Input: part model. Units: mm. Frame: model coordinates. Give positions to 0.01 mm unless a question says otherwise; leave off trailing zeros. Write each loop counter-clockwise with the first axis right and the second up, starting at its lowest first coordinate (ties: lowest second). Pieces come first, ordered by that corner, then holes. Notation, with made-up numbers: (39, -35.75) -> (82, -35.75) arc R24 cw to (82, -3.75) -> close; hole circle Ø1 at (-15.5, -16.5). An arc over 180 degrees is marked (long way). Answer as a JSON object with one key per item and string values. Group by question number.
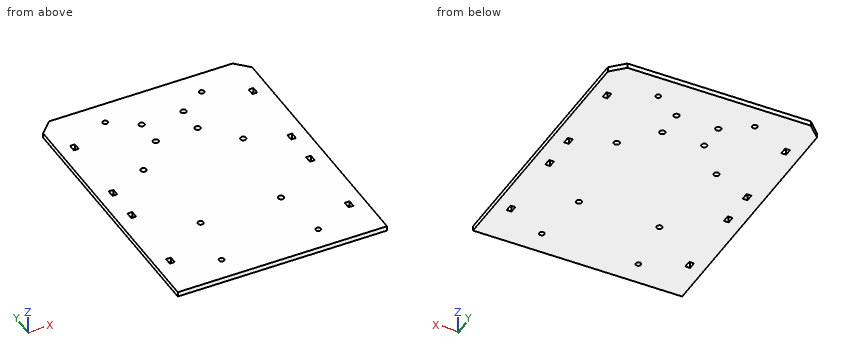
from build123d import *

# Parameters (mm, degrees)
SKETCH_1_R      = 1.6
SKETCH_1_R_2    = 1.75
SKETCH_1_W      = 3
SKETCH_1_H      = 4.6
EXTRUDE_1_DEPTH = 3


with BuildPart() as part:
    # ｽｹｯﾁ1 → ﾎﾞｽ - 押し出し1 (new body)
    with BuildSketch(Plane.XY):
        Polygon((0, 162), (8, 170), (122, 170), (130, 162), (130, 0), (0, 0), align=None)
        with Locations((35, 155)):
            Circle(SKETCH_1_R, mode=Mode.SUBTRACT)
        with Locations((95, 155)):
            Circle(SKETCH_1_R, mode=Mode.SUBTRACT)
        with Locations((35, 15)):
            Circle(SKETCH_1_R, mode=Mode.SUBTRACT)
        with Locations((95, 15)):
            Circle(SKETCH_1_R, mode=Mode.SUBTRACT)
        with Locations((34, 107)):
            Circle(SKETCH_1_R_2, mode=Mode.SUBTRACT)
        with Locations((96, 107)):
            Circle(SKETCH_1_R_2, mode=Mode.SUBTRACT)
        with Locations((40, 50)):
            Circle(SKETCH_1_R_2, mode=Mode.SUBTRACT)
        with Locations((90, 50)):
            Circle(SKETCH_1_R_2, mode=Mode.SUBTRACT)
        with Locations((52, 144)):
            Circle(SKETCH_1_R_2, mode=Mode.SUBTRACT)
        with Locations((78, 144)):
            Circle(SKETCH_1_R_2, mode=Mode.SUBTRACT)
        with Locations((52, 127)):
            Circle(SKETCH_1_R_2, mode=Mode.SUBTRACT)
        with Locations((78, 127)):
            Circle(SKETCH_1_R_2, mode=Mode.SUBTRACT)
        with Locations((9.5, 142.7)):
            Rectangle(SKETCH_1_W, SKETCH_1_H, mode=Mode.SUBTRACT)
        with Locations((120.5, 142.7)):
            Rectangle(SKETCH_1_W, SKETCH_1_H, mode=Mode.SUBTRACT)
        with Locations((9.5, 27.3)):
            Rectangle(SKETCH_1_W, SKETCH_1_H, mode=Mode.SUBTRACT)
        with Locations((120.5, 27.3)):
            Rectangle(SKETCH_1_W, SKETCH_1_H, mode=Mode.SUBTRACT)
        with Locations((9.5, 96.3)):
            Rectangle(SKETCH_1_W, SKETCH_1_H, mode=Mode.SUBTRACT)
        with Locations((120.5, 96.3)):
            Rectangle(SKETCH_1_W, SKETCH_1_H, mode=Mode.SUBTRACT)
        with Locations((9.5, 73.7)):
            Rectangle(SKETCH_1_W, SKETCH_1_H, mode=Mode.SUBTRACT)
        with Locations((120.5, 73.7)):
            Rectangle(SKETCH_1_W, SKETCH_1_H, mode=Mode.SUBTRACT)
    extrude(amount=EXTRUDE_1_DEPTH)


solid = part.part
1. Section B-B (x = 52). Return the cut outline in (y, z), plus the area to 3 significant figures.
2. Contact query for a flat-ended pin moving along its axis: pin 1 Ø2 at (x, y) = (96, 107) entering from -Z. Output: stop coordinate, or through.
3. Section A-A (x = 90). Return the cut outline in (y, z), plus the area to 4 significant figures.
4. Section C-C (y = 127). Return the cut outline in (x, z).
5. Line query: line 1 (X direction, y = 71.5, z = 0.5); line 2 (X direction, y = 107, z = 2.15); line 3 (Y direction, x = 90, z = 1.6). Output: solid intervals per line, ascending.
Working result:
{
 "1": {"outline": "(0, 0) -> (125.25, 0) -> (125.25, 3) -> (0, 3) -> close; (128.75, 0) -> (142.25, 0) -> (142.25, 3) -> (128.75, 3) -> close; (145.75, 0) -> (170, 0) -> (170, 3) -> (145.75, 3) -> close", "area": "489 mm^2"},
 "2": {"pin 1": "passes through"},
 "3": {"outline": "(0, 0) -> (48.25, 0) -> (48.25, 3) -> (0, 3) -> close; (51.75, 0) -> (170, 0) -> (170, 3) -> (51.75, 3) -> close", "area": "499.5 mm^2"},
 "4": {"outline": "(0, 0) -> (50.25, 0) -> (50.25, 3) -> (0, 3) -> close; (53.75, 0) -> (76.25, 0) -> (76.25, 3) -> (53.75, 3) -> close; (79.75, 0) -> (130, 0) -> (130, 3) -> (79.75, 3) -> close"},
 "5": {"line 1": "x = 0 to 8, 11 to 119, 122 to 130", "line 2": "x = 0 to 32.25, 35.75 to 94.25, 97.75 to 130", "line 3": "y = 0 to 48.25, 51.75 to 170"}
}
